from build123d import *
from build123d.topology import SkipClean

# Parameters (mm, degrees)
SKETCH1_R           = 7.5
SKETCH1_R_2         = 4
BOSS_EXTRUDE2_DEPTH = 15
CUT_EXTRUDE3_DEPTH  = 486.130191019
FILLET1_R           = 4
CUT_EXTRUDE8_DEPTH  = 10
SKETCH16_R          = 46.355085109
CUT_EXTRUDE9_DEPTH  = 10
FILLET6_R           = 3
FILLET7_R           = 3


with BuildPart() as part:
    # Sketch1 → Boss-Extrude2 (new, symmetric)
    with BuildSketch(Plane(origin=(1165, 0, 0), x_dir=(0, 0, -1), z_dir=(1, 0, 0))):
        with BuildLine():
            Line((-401.950614401, -252.930875731), (-341.032402001, -244.870391996))
            ThreePointArc((-341.032402001, -244.870391996), (-328, -230), (-341.032402001, -215.129608004))
            Line((-341.032402001, -215.129608004), (-401.950614401, -207.069124269))
            ThreePointArc((-401.950614401, -207.069124269), (-407.498189204, -208.384390135), (-410.761140001, -213.059715))
            ThreePointArc((-410.761140001, -213.059715), (-412.846584384, -230), (-410.761140001, -246.940285))
            ThreePointArc((-410.761140001, -246.940285), (-407.498189204, -251.615609865), (-401.950614401, -252.930875731))
        make_face()
        with Locations((-343, -230)):
            Circle(SKETCH1_R, mode=Mode.SUBTRACT)
        with Locations((-403, -215)):
            Circle(SKETCH1_R_2, mode=Mode.SUBTRACT)
        with Locations((-403, -245)):
            Circle(SKETCH1_R_2, mode=Mode.SUBTRACT)
    extrude(amount=BOSS_EXTRUDE2_DEPTH, both=True)

    # Sketch3 → Cut-Extrude3 (cut, through all)
    with BuildSketch(Plane.ZY.offset(-1150)):
        with BuildLine():
            Line((386.199035454, -246.8118188), (356.915169615, -242.937080606))
            Line((356.915169615, -242.937080606), (351.667017329, -242.242663543))
            ThreePointArc((351.667017329, -242.242663543), (358, -230), (351.667017329, -217.757336457))
            Line((351.667017329, -217.757336457), (356.915169615, -217.062919394))
            Line((356.915169615, -217.062919394), (386.199035454, -213.1881812))
            ThreePointArc((386.199035454, -213.1881812), (389.355085109, -230), (386.199035454, -246.8118188))
        make_face()
    extrude(amount=-CUT_EXTRUDE3_DEPTH, mode=Mode.SUBTRACT)

    # Fillet1
    fillet1_edges = [part.edges().sort_by_distance(p)[0] for p in [
        (1165, -246.8118188, 386.199035454),
        (1165, -242.242663543, 351.667017329),
        (1165, -217.757336457, 351.667017329),
        (1165, -213.1881812, 386.199035454),
    ]]
    fillet(fillet1_edges, radius=FILLET1_R)

    # Sketch14 → Cut-Extrude8 (cut, symmetric)
    with BuildSketch(Plane(origin=(1165, 0, 0), x_dir=(0, 0, -1), z_dir=(1, 0, 0))):
        with BuildLine():
            Line((-374.476194015, -186.80167911), (-394.628690595, -182.957214607))
            ThreePointArc((-394.628690595, -182.957214607), (-412.839050853, -231.025829466), (-393.224741594, -278.538857444))
            Line((-393.224741594, -278.538857444), (-380.9384348, -267.649978517))
            ThreePointArc((-380.9384348, -267.649978517), (-396.279541596, -225.741342376), (-374.476194015, -186.80167911))
        make_face()
    extrude(amount=CUT_EXTRUDE8_DEPTH, both=True, mode=Mode.SUBTRACT)

    # Sketch16 → Cut-Extrude9 (cut, symmetric)
    with SkipClean():  # the faces are left unmerged after this step: merging them gives an invalid solid
        with BuildSketch(Plane(origin=(1165, 0, 0), x_dir=(0, 0, -1), z_dir=(1, 0, 0))):
            with Locations((-343, -230)):
                Circle(SKETCH16_R)
        extrude(amount=CUT_EXTRUDE9_DEPTH, both=True, mode=Mode.SUBTRACT)

    # Fillet6
    fillet6_edges = [part.edges().sort_by_distance(p)[0] for p in [
        (1165, -208.400223767, 391.890647205),
        (1165, -251.599776233, 391.890647205),
    ]]
    fillet(fillet6_edges, radius=FILLET6_R)

    # Fillet7
    fillet7_edges = [part.edges().sort_by_distance(p)[0] for p in [
        (1165, -250.623789579, 384.514494082),
        (1165, -209.376210421, 384.514494082),
    ]]
    fillet(fillet7_edges, radius=FILLET7_R)


solid = part.part
Here's how the part is built. I have some questions about the finished solid (model axes, mm). A direction names the side the tool comes from. Give positions to 0.01 mm unless a question says otherwise; leave off trailing zeros. Order: outer loops, then holes, each group sorted by start corner. A loop starts at its lowest first (then second) coordinate and runs counter-clockwise, first axis right, second up. Notation, with made-up numbers: (13, 62) -> (29, 62) arc R17 cw to (29, 77) -> close; hole circle Ø7 at (15.5, 10.5). An arc over 180 degrees is marked (long way). One line per item, written item: value. Start each with the question number.
1. Imagine slicing it at C-C, the plane z = 348. List the corners of the cut face in (x, y) for me.
2. We'd pull the mould along X, two halves only. Please class faces 1 (the face through (1180, -230, 390)), 2 (the face through (1177.54, -208.34, 407.43)), 3 (the face through (1165.1, -210.3, 386.3)): released by +X, released by -X, zero draft, split by the parting line, or undercut.
3. Imagine slicing it at A-A, the plane z = 403. List the corners of the cut face in (x, y) for me.
4. I need wall thicknesses on probe 1 along Y at (x, z) = (1176.1, 403); probe 2 along Z at (x, y) = (1152.45, -230); probe 3 along Y at (x, z) = (1178, 405). Which ranges of each line are inside material? Lowest first, please. Write a range as from..to.
5. For faces 4 (the face through (1165.1, -249.7, 386.3)), 5 (the face through (1177.535, -245.806, 385.622)), 6 (the face through (1153, -230, 328)), which set-ups out of +Z, -Z, +X, -X, +Y, -Y let a thin tool reach every point of the face, with its end or its side?
6. Imagine slicing it at B-B, the plane y = -230. List the corners of the cut face in (x, z) for me, plus the area to 3 significant figures.
7. Will these pins go through, and if not, where does the flat tip stop? pin 1 Ø8 at (x, z) = (1156.5, 398.5) entering from -Y; pin 2 Ø10 at (x, y) = (1167.5, -233.5) entering from -Z; pin 3 Ø9 at (y, z) = (-230, 343) entering from -X; pin 4 Ø10 at (x, z) = (1174.5, 393.5) entering from +Y.
8. Imagine slicing it at D-D, the plane x = 1171.5. List the corners of the cut face in (y, z) for me.
Values follow:
1. outline: (1150, -245.79) -> (1155, -245.79) -> (1155, -235.59) -> (1150, -235.59) -> close; (1150, -224.41) -> (1155, -224.41) -> (1155, -214.21) -> (1150, -214.21) -> close; (1175, -245.79) -> (1180, -245.79) -> (1180, -235.59) -> (1175, -235.59) -> close; (1175, -224.41) -> (1180, -224.41) -> (1180, -214.21) -> (1175, -214.21) -> close
2. face 1: released by +X
2. face 2: zero draft
2. face 3: undercut
3. outline: (1150, -253) -> (1155, -253) -> (1155, -249) -> (1150, -249) -> close; (1150, -241) -> (1155, -241) -> (1155, -219) -> (1150, -219) -> close; (1150, -211) -> (1155, -211) -> (1155, -207) -> (1150, -207) -> close; (1175, -253) -> (1180, -253) -> (1180, -249) -> (1175, -249) -> close; (1175, -241) -> (1180, -241) -> (1180, -219) -> (1175, -219) -> close; (1175, -211) -> (1180, -211) -> (1180, -207) -> (1175, -207) -> close
4. probe 1: y = -253..-249, -241..-219, -211..-207
4. probe 2: z = 328..335.5, 350.5..358, 389.36..412.85
4. probe 3: y = -252.75..-248.46, -241.54..-218.46, -211.54..-207.25
5. face 4: -Z
5. face 5: +X, -X
5. face 6: -Z, +X, -X
6. outline: (1150, 328) -> (1155, 328) -> (1155, 335.5) -> (1150, 335.5) -> close; (1150, 350.5) -> (1155, 350.5) -> (1155, 358) -> (1150, 358) -> close; (1150, 389.36) -> (1180, 389.36) -> (1180, 412.85) -> (1175, 412.85) -> (1175, 396.45) -> (1155, 396.45) -> (1155, 412.85) -> (1150, 412.85) -> close; (1175, 328) -> (1180, 328) -> (1180, 335.5) -> (1175, 335.5) -> close; (1175, 350.5) -> (1180, 350.5) -> (1180, 358) -> (1175, 358) -> close
6. area: 527 mm2
7. pin 1: stops at y = -252.96
7. pin 2: stops at z = 388.57
7. pin 3: passes through
7. pin 4: stops at y = -207.53
8. outline: (-251.3, 389.61) -> (-251.15, 388.49) arc R3 ccw to (-247.07, 386.1) arc R46.36 cw to (-212.93, 386.1) arc R3 ccw to (-208.85, 388.49) -> (-208.7, 389.61) arc R3 ccw to (-210.59, 392.8) arc R53.45 ccw to (-249.41, 392.8) arc R3 ccw to start
